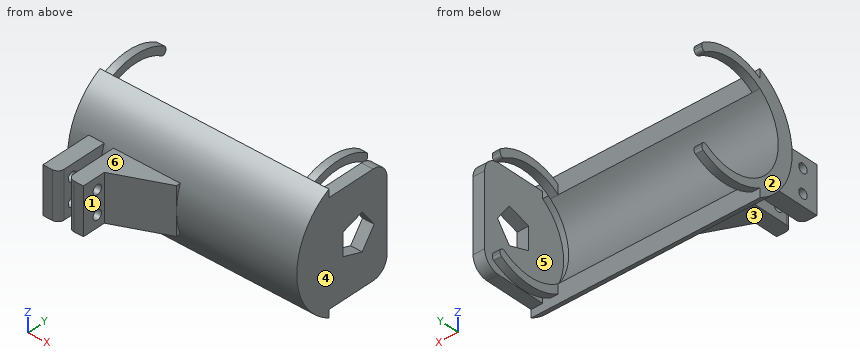
```python
from build123d import *

# Parameters (mm, degrees)
BOSS_EXTRUDE1_DEPTH   = 70
BOSS_EXTRUDE2_START   = -5
BOSS_EXTRUDE2_DEPTH   = 5
BOSS_EXTRUDE3_START   = 7.5
BOSS_EXTRUDE3_DEPTH   = 7.5
BOSS_EXTRUDE4_DEPTH   = 15
BOSS_EXTRUDE4_2_DEPTH = 15
BOSS_EXTRUDE6_REACH   = 109.8
SKETCH5_W             = 43
SKETCH5_H             = 30
SKETCH5_W_2           = 10
CUT_EXTRUDE1_REACH    = 161.406
SKETCH6_R             = 3
SKETCH7_R             = 35
CUT_EXTRUDE2_DEPTH    = 5
LPATTERN1_COUNT       = 2
LPATTERN1_PITCH       = 130
FILLET1_R             = 2
CUT_EXTRUDE3_REACH    = 164.413


with BuildPart() as part:
    # Sketch1 → Boss-Extrude1 (new, symmetric)
    with BuildSketch(Plane(origin=(0, 0, 0), x_dir=(0, 0, -1), z_dir=(1, 0, 0))):
        with BuildLine():
            Line((-38.065732621, -20), (-26.248809497, -20))
            ThreePointArc((-26.248809497, -20), (0, -33), (26.248809497, -20))
            Line((26.248809497, -20), (38.065732621, -20))
            ThreePointArc((38.065732621, -20), (0, -43), (-38.065732621, -20))
        make_face()
    extrude(amount=BOSS_EXTRUDE1_DEPTH, both=True)

    # Sketch2 → Boss-Extrude2 (add)
    with BuildSketch(Plane(origin=(70, 0, 0), x_dir=(0, 0, -1), z_dir=(1, 0, 0)).offset(BOSS_EXTRUDE2_START)):
        with BuildLine():
            Line((-31.304951685, 21.540659229), (-25, 21.540659229))
            ThreePointArc((-25, 21.540659229), (0, -33), (25, 21.540659229))
            Line((25, 21.540659229), (31.304951685, 21.540659229))
            ThreePointArc((31.304951685, 21.540659229), (0, -38), (-31.304951685, 21.540659229))
        make_face()
    boss_extrude2 = extrude(amount=-BOSS_EXTRUDE2_DEPTH)

    # Sketch3 → Boss-Extrude3 (add)
    with BuildSketch(Plane(origin=(70, 0, 0), x_dir=(0, 0, -1), z_dir=(1, 0, 0)).offset(BOSS_EXTRUDE3_START)):
        with BuildLine():
            Line((-33, -20), (-33, 11.540659229))
            ThreePointArc((-33, 11.540659229), (-30.071067812, 18.61172704), (-23, 21.540659229))
            Line((-23, 21.540659229), (23, 21.540659229))
            ThreePointArc((23, 21.540659229), (30.071067812, 18.61172704), (33, 11.540659229))
            Line((33, 11.540659229), (33, -20))
            Line((33, -20), (38.065732621, -20))
            ThreePointArc((38.065732621, -20), (0, -43), (-38.065732621, -20))
            Line((-38.065732621, -20), (-33, -20))
        make_face()
    extrude(amount=-BOSS_EXTRUDE3_DEPTH)

    # Sketch5 → Boss-Extrude6 (add, up to next)
    with BuildSketch(Plane(origin=(0, -43, 0), x_dir=(1, 0, 0), z_dir=(0, 1, 0)), mode=Mode.PRIVATE) as boss_extrude6_sk1:
        with Locations((-21.5, 0)):
            Rectangle(SKETCH5_W, SKETCH5_H)
    boss_extrude6_tool1 = extrude(boss_extrude6_sk1.sketch, amount=BOSS_EXTRUDE6_REACH, mode=Mode.PRIVATE) - part.part
    # Sketch5 → Boss-Extrude6 (add, up to next)
    with BuildSketch(Plane(origin=(0, -43, 0), x_dir=(1, 0, 0), z_dir=(0, 1, 0)), mode=Mode.PRIVATE) as boss_extrude6_sk2:
        with Locations((-54, 0)):
            Rectangle(SKETCH5_W_2, SKETCH5_H)
    boss_extrude6_tool2 = extrude(boss_extrude6_sk2.sketch, amount=BOSS_EXTRUDE6_REACH, mode=Mode.PRIVATE) - part.part


with BuildPart() as body_2:
    # Sketch4 → Boss-Extrude4 (new, symmetric)
    with BuildSketch(Plane.XY):
        with BuildLine():
            Line((-49, -43), (-49, -69))
            ThreePointArc((-49, -69), (-50.171572875, -71.828427125), (-53, -73))
            Line((-53, -73), (-59, -73))
            Line((-59, -73), (-59, -43))
            Line((-59, -43), (-49, -43))
        make_face()
    extrude(amount=BOSS_EXTRUDE4_DEPTH, both=True)


with BuildPart() as body_3:
    # Sketch4 → Boss-Extrude4 2 (new, symmetric)
    with BuildSketch(Plane.XY):
        with BuildLine():
            Line((-33, -43), (-43, -43))
            Line((-43, -43), (-43, -69))
            ThreePointArc((-43, -69), (-41.828427125, -71.828427125), (-39, -73))
            Line((-39, -73), (-33, -73))
            Line((-33, -73), (-33, -58))
            Line((-33, -58), (0, -43))
            Line((0, -43), (-33, -43))
        make_face()
    extrude(amount=BOSS_EXTRUDE4_2_DEPTH, both=True)


with BuildPart() as part_1:
    add(part.part)

    add(body_2.part)  # Boss-Extrude6 merges body 2

    add(body_3.part)  # Boss-Extrude6 merges body 3
    add(boss_extrude6_tool1.solids().sort_by_distance((-21.5, -43, 0))[0])
    add(boss_extrude6_tool1.solids().sort_by_distance((-21.5, -43, 0))[1])
    add(boss_extrude6_tool2.solids().sort_by_distance((-54, -43, 0))[0])
    add(boss_extrude6_tool2.solids().sort_by_distance((-54, -43, 0))[1])

    # Cut-Extrude1: up to this face of the body (flat: up to its plane)
    cut_extrude1_end = Plane(part_1.part.faces().sort_by_distance((-33, -65.5, 0))[0])
    # Sketch6 → Cut-Extrude1 (cut, up to the picked face)
    with BuildSketch(Plane.ZY.offset(59), mode=Mode.PRIVATE) as cut_extrude1_sk1:
        with Locations((-7.5, -63)):
            Circle(SKETCH6_R)
    cut_extrude1_tool1 = split(extrude(cut_extrude1_sk1.sketch, amount=-CUT_EXTRUDE1_REACH, mode=Mode.PRIVATE), bisect_by=cut_extrude1_end, keep=Keep.BOTH, mode=Mode.PRIVATE)
    # Sketch6 → Cut-Extrude1 (cut, up to the picked face)
    with BuildSketch(Plane.ZY.offset(59), mode=Mode.PRIVATE) as cut_extrude1_sk2:
        with Locations((7.5, -63)):
            Circle(SKETCH6_R)
    cut_extrude1_tool2 = split(extrude(cut_extrude1_sk2.sketch, amount=-CUT_EXTRUDE1_REACH, mode=Mode.PRIVATE), bisect_by=cut_extrude1_end, keep=Keep.BOTH, mode=Mode.PRIVATE)
    add(cut_extrude1_tool1.solids().sort_by(Axis((-59, -63, -7.5), (1, 0, 0)))[0], mode=Mode.SUBTRACT)
    add(cut_extrude1_tool2.solids().sort_by(Axis((-59, -63, 7.5), (1, 0, 0)))[0], mode=Mode.SUBTRACT)

    # Sketch7 → Cut-Extrude2 (cut)
    with BuildSketch(Plane.ZY.offset(-70)):
        Circle(SKETCH7_R)
    extrude(amount=CUT_EXTRUDE2_DEPTH, mode=Mode.SUBTRACT)

    # LPattern1: Boss-Extrude2 ×2
    with Locations(*[(-i * LPATTERN1_PITCH, 0, 0) for i in range(1, LPATTERN1_COUNT)]):
        add(boss_extrude2)

    # Fillet1
    fillet1_edges = [part_1.edges().sort_by_distance(p)[0] for p in [
        (62.5, 21.540659229, 25),
        (62.5, 21.540659229, -31.304951685),
        (-67.5, 21.540659229, 25),
        (-67.5, 21.540659229, -31.304951685),
        (-67.5, 21.540659229, -25),
        (-67.5, 21.540659229, 31.304951685),
        (62.5, 21.540659229, -25),
        (62.5, 21.540659229, 31.304951685),
    ]]
    fillet(fillet1_edges, radius=FILLET1_R)

    # Sketch8 → Cut-Extrude3 (cut, up to next)
    with BuildSketch(Plane.ZY.offset(-70), mode=Mode.PRIVATE) as cut_extrude3_sk1:
        Polygon((0, 12.360679775), (-11.755705046, 3.819660113), (-7.26542528, -10), (7.26542528, -10), (11.755705046, 3.819660113), align=None)
    cut_extrude3_tool1 = extrude(cut_extrude3_sk1.sketch, amount=-CUT_EXTRUDE3_REACH, mode=Mode.PRIVATE) & part_1.part
    add(cut_extrude3_tool1.solids().sort_by_distance((70, 0, 0))[0], mode=Mode.SUBTRACT)


solid = part_1.part
```
For this review, take the finished solid that the model builds, in its own axes (mm). Face numbers are marked on the shaded views. A direction names the side the tool comes from. Round coordinates to 2 decimals unless told otherwise and drop trailing zeros. Write each loop counter-clockwise with the first axis right and the second up, starting at its lowest first coordinate (ties: lowest second). Pieces come first, ordered by that corner, then holes. Notation, with made-up numbers: (12, 41) -> (16, 41) arc R21 ccw to (16, 47) -> close; hole circle Ø3 at (51.25, 32). An arc over 180 degrees is marked (long way). Use one line per item in the form item = value.
1) To check wall thickness, follow L1, parallel to X at y = -57.5, z = -6; L2, parallel to X at y = -4.5, z = -29; L3, parallel to X at y = -52.5, z = 3.5. State the ranges of each line that lie inside material, in increasing order. Write a range as from..to.
Found:
L1 = -59..-49, -43..-31.9
L2 = 70..77.5
L3 = -59..-49, -43..-20.9
2) Take a section at D-D, the plane x = -28. Write out the cut boundary in (y, z).
Found:
outline = (-55.73, -15) -> (-40.3, -15) arc R43 ccw to (-20, -38.07) -> (-20, -26.25) arc R33 cw to (-20, 26.25) -> (-20, 38.07) arc R43 ccw to (-40.3, 15) -> (-55.73, 15) -> close
3) Take a section at A-A, the plane y = 7. Write out the cut boundary in (x, z), and give its area (3 significant figures).
Found:
outline = (-70, -37.35) -> (-65, -37.35) -> (-65, -32.25) -> (-70, -32.25) -> close; (-70, 32.25) -> (-65, 32.25) -> (-65, 37.35) -> (-70, 37.35) -> close; (60, -37.35) -> (65, -37.35) -> (65, -32.25) -> (60, -32.25) -> close; (60, 32.25) -> (65, 32.25) -> (65, 37.35) -> (60, 37.35) -> close; (70, -33) -> (77.5, -33) -> (77.5, -7.38) -> (70, -7.38) -> close; (70, 7.38) -> (77.5, 7.38) -> (77.5, 33) -> (70, 33) -> close
area = 486 mm2
4) Clearance check with flat-ended pins moving along their axes: pin 1 (2 mm diameter, centred on x = 75, y = 2, fed in from -Z); pin 2 (12 mm diameter, centred on x = 32.5, y = -34, fed in from +Z); pin 3 (6 mm diameter, centred on x = -10.5, z = 31, fed in from +Y); pin 4 (3.5 mm diameter, centred on y = -63, z = -7.5, fed in from -X). State where each tip first meets the part, or that it passes through.
Found:
pin_1 = -33
pin_2 = 32.63
pin_3 = -20
pin_4 = through
5) Take a section at C-C, the plane y = -28.5. Write out the cut boundary in (x, z).
Found:
outline = (-70, -32.2) -> (77.5, -32.2) -> (77.5, 32.2) -> (-70, 32.2) -> (-70, 16.64) -> (65, 16.64) -> (65, 20.32) -> (70, 20.32) -> (70, -20.32) -> (65, -20.32) -> (65, -16.64) -> (-70, -16.64) -> close
6) Tool access review of the marked faces 1, 2 and 3: name each direction out of +Z, -Z, +X, -X, +Y, -Y from which nothing blocks a thin tool from reaching the whole face with its end or side.
Found:
face_1 = +Z, -Z, +X, -Y
face_2 = +Z, -Z, -X, +Y, -Y
face_3 = -Z, +X, -X, -Y
7) Mouldability with a two-part tool opening along Z and no side actions: class the marked faces 4, 5 and 6 as +Z half, -Z half, draft (parallel to the pull), parting line (faces both ways), or undercut.
Found:
face_4 = draft
face_5 = undercut
face_6 = +Z half
